```python
from build123d import *
from build123d.topology import SkipClean

# Parameters (mm, degrees)
SKETCH1_W           = 30
SKETCH1_H           = 59
SKETCH1_R           = 7
BOSS_EXTRUDE1_DEPTH = 30
CUT_EXTRUDE1_START  = -14.5
SKETCH2_W           = 30
SKETCH2_H           = 2
CUT_EXTRUDE1_DEPTH  = 4
BOSS_EXTRUDE2_START = 12
SKETCH4_W           = 45
SKETCH4_H           = 59
SKETCH4_R           = 7
BOSS_EXTRUDE2_DEPTH = 12
SKETCH5_R           = 8
CUT_EXTRUDE3_DEPTH  = 8.5
SKETCH8_R           = 10
CUT_EXTRUDE5_DEPTH  = 3.5
BOSS_EXTRUDE4_START = 1.5
BOSS_EXTRUDE4_DEPTH = 1.5
SKETCH12_R          = 6
CUT_EXTRUDE7_DEPTH  = 22
CHAMFER1_SIZE       = 2
MOVE_FACE1_BY       = 1
SKETCH16_W          = 1
SKETCH16_H          = 8
BOSS_EXTRUDE5_DEPTH = 15
SKETCH14_R          = 2.25
CUT_EXTRUDE9_DEPTH  = 70.083283072
BOSS_EXTRUDE6_DEPTH = 20
SKETCH18_R          = 5
CUT_EXTRUDE10_DEPTH = 3
SKETCH19_R          = 2.25
CUT_EXTRUDE11_DEPTH = 81.873357789
SKETCH20_R          = 5
CUT_EXTRUDE12_DEPTH = 7
CHAMFER2_SIZE       = 8
CUT_EXTRUDE13_DEPTH = 2
SKETCH22_R          = 3.3
CUT_EXTRUDE14_DEPTH = 15
CUT_EXTRUDE15_START = -3
CUT_EXTRUDE15_DEPTH = 7
SKETCH24_W          = 8
SKETCH24_H          = 4
SKETCH24_W_2        = 4
SKETCH24_H_2        = 8
BOSS_EXTRUDE7_DEPTH = 4
CUT_EXTRUDE16_START = -31.5
CUT_EXTRUDE16_DEPTH = 31.5


with BuildPart() as part:
    # Sketch1 → Boss-Extrude1 (new body)
    with BuildSketch(Plane.XY):
        with Locations((0, -15)):
            Rectangle(SKETCH1_W, SKETCH1_H)
        Circle(SKETCH1_R, mode=Mode.SUBTRACT)
    extrude(amount=-BOSS_EXTRUDE1_DEPTH)

    # Sketch2 → Cut-Extrude1 (cut, symmetric)
    with BuildSketch(Plane.XZ.offset(44.5).offset(CUT_EXTRUDE1_START)):
        with Locations((0, -29)):
            Rectangle(SKETCH2_W, SKETCH2_H)
    extrude(amount=CUT_EXTRUDE1_DEPTH, both=True, mode=Mode.SUBTRACT)

    # Sketch4 → Boss-Extrude2 (add)
    with BuildSketch(Plane.XY.offset(BOSS_EXTRUDE2_START)):
        with Locations((7.5, -15)):
            Rectangle(SKETCH4_W, SKETCH4_H)
        Circle(SKETCH4_R, mode=Mode.SUBTRACT)
    extrude(amount=-BOSS_EXTRUDE2_DEPTH)

    # Sketch5 → Cut-Extrude3 (cut)
    with BuildSketch(Plane.XY.offset(12)):
        Circle(SKETCH5_R)
    extrude(amount=-CUT_EXTRUDE3_DEPTH, mode=Mode.SUBTRACT)

    # Sketch8 → Cut-Extrude5 (cut)
    with BuildSketch(Plane.XY.offset(12)):
        Circle(SKETCH8_R)
    extrude(amount=-CUT_EXTRUDE5_DEPTH, mode=Mode.SUBTRACT)

    # Sketch11 → Boss-Extrude4 (add)
    with SkipClean():  # the faces are left unmerged after this step: merging them gives an invalid solid
        with BuildSketch(Plane.XY.offset(12).offset(BOSS_EXTRUDE4_START)):
            with BuildLine():
                Line((30, 14.5), (8, 14.5))
                Line((8, 14.5), (8, 6))
                ThreePointArc((8, 6), (10, 0), (8, -6))
                Line((8, -6), (8, -44.5))
                Line((8, -44.5), (30, -44.5))
                Line((30, -44.5), (30, 14.5))
            make_face()
        extrude(amount=-BOSS_EXTRUDE4_DEPTH)

    # Sketch12 → Cut-Extrude7 (cut)
    with SkipClean():  # the faces are left unmerged after this step: merging them gives an invalid solid
        with BuildSketch(Plane(origin=(30, 0, 0), x_dir=(0, 0, -1), z_dir=(1, 0, 0))):
            with Locations((-15, -19)):
                Circle(SKETCH12_R)
        extrude(amount=-CUT_EXTRUDE7_DEPTH, mode=Mode.SUBTRACT)

    # Chamfer1
    # the kernel refuses this chamfer: 2 mm, written as the material it adds along each edge
    with BuildSketch(Plane(origin=(8, -19.052786447, 12), x_dir=(-0.9996219169112968, 0, -0.027495876610586487), z_dir=(0, -1, 0))) as chamfer1_piece_1_section:
        Polygon((CHAMFER1_SIZE * 0.999621916911, -CHAMFER1_SIZE * 0.0274958766106), (-CHAMFER1_SIZE * 0.0274958766106, -CHAMFER1_SIZE * 0.999621916911), (0, 0), align=None)
    chamfer1_piece_1 = extrude(amount=25.447213553, mode=Mode.PRIVATE)
    chamfer1_piece_1 = chamfer1_piece_1 - Plane(origin=(7.298262976, -19, 15), x_dir=(0, 0, -1), z_dir=(1, 0, 0)) * Cylinder(6, 59, mode=Mode.PRIVATE)
    chamfer1_piece_1 = split(chamfer1_piece_1, bisect_by=Plane(origin=(7.298262976, -34.489945177, 13.5), z_dir=(0, 0, -1)), keep=Keep.TOP, mode=Mode.PRIVATE)
    add(chamfer1_piece_1)
    with BuildSketch(Plane(origin=(8, 14.5, 12), x_dir=(-0.9996219169112968, 0, -0.027495876610586487), z_dir=(0, -1, 0))) as chamfer1_piece_2_section:
        Polygon((CHAMFER1_SIZE * 0.999621916911, -CHAMFER1_SIZE * 0.0274958766106), (-CHAMFER1_SIZE * 0.0274958766106, -CHAMFER1_SIZE * 0.999621916911), (0, 0), align=None)
    chamfer1_piece_2 = extrude(amount=13.643365976, mode=Mode.PRIVATE)
    chamfer1_piece_2 = chamfer1_piece_2 - Plane(origin=(0, 0, 12.610971558), x_dir=(1, 0, 0), z_dir=(0, 0, 1)) * Cylinder(10, 36, mode=Mode.PRIVATE)
    chamfer1_piece_2 = split(chamfer1_piece_2, bisect_by=Plane(origin=(7.329577736, 10.634975656, 13.5), z_dir=(0, 0, -1)), keep=Keep.TOP, mode=Mode.PRIVATE)
    add(chamfer1_piece_2)
    with BuildSketch(Plane(origin=(8, -0.856634024, 12), x_dir=(-0.9996219169112968, 0, -0.027495876610586487), z_dir=(0, -1, 0))) as chamfer1_piece_3_section:
        Polygon((CHAMFER1_SIZE * 0.999621916911, -CHAMFER1_SIZE * 0.0274958766106), (-CHAMFER1_SIZE * 0.0274958766106, -CHAMFER1_SIZE * 0.999621916911), (0, 0), align=None)
    chamfer1_piece_3 = extrude(amount=18.090579529, mode=Mode.PRIVATE)
    chamfer1_piece_3 = chamfer1_piece_3 - Plane(origin=(7.328722349, -19, 15), x_dir=(0, 0, -1), z_dir=(1, 0, 0)) * Cylinder(6, 45, mode=Mode.PRIVATE)
    chamfer1_piece_3 = chamfer1_piece_3 - Plane(origin=(0, 0, 12.602221716), x_dir=(1, 0, 0), z_dir=(0, 0, 1)) * Cylinder(10, 45, mode=Mode.PRIVATE)
    chamfer1_piece_3 = split(chamfer1_piece_3, bisect_by=Plane(origin=(7.328722349, -10.144229593, 13.5), z_dir=(0, 0, -1)), keep=Keep.TOP, mode=Mode.PRIVATE)
    add(chamfer1_piece_3)

    # Move Face1: a face moved outward by 1.0
    extrude(part.faces().sort_by_distance((8, -19, 10.769879029))[0], amount=MOVE_FACE1_BY, dir=(1, 0, 0))

    # Sketch16 → Boss-Extrude5 (add)
    with BuildSketch(Plane(origin=(30, 0, 0), x_dir=(0, 0, -1), z_dir=(1, 0, 0))):
        with Locations((0.5, 0)):
            Rectangle(SKETCH16_W, SKETCH16_H)
        with Locations((0.5, -30)):
            Rectangle(SKETCH16_W, SKETCH16_H)
    extrude(amount=-BOSS_EXTRUDE5_DEPTH)

    # Sketch14 → Cut-Extrude9 (cut, through all)
    with BuildSketch(Plane.XY.offset(13.5)):
        with Locations((22.5, 0)):
            Circle(SKETCH14_R)
        with Locations((22.5, -30)):
            Circle(SKETCH14_R)
    extrude(amount=-CUT_EXTRUDE9_DEPTH, mode=Mode.SUBTRACT)

    # Sketch18 → Cut-Extrude10 (cut)
    with BuildSketch(Plane.XY.offset(13.5)):
        with Locations((22.5, 0)):
            Circle(SKETCH18_R)
    extrude(amount=-CUT_EXTRUDE10_DEPTH, mode=Mode.SUBTRACT)

    # Sketch21 → Cut-Extrude13 (cut)
    with BuildSketch(Plane(origin=(15, 0, 0), x_dir=(0, 0, -1), z_dir=(1, 0, 0))):
        Polygon((0, 9), (10, 9), (10, -9), (0, -9), (0, -4), (1, -4), (1, 4), (0, 4), align=None)
        Polygon((0, -21), (10, -21), (10, -39), (0, -39), (0, -34), (1, -34), (1, -26), (0, -26), align=None)
    extrude(amount=-CUT_EXTRUDE13_DEPTH, mode=Mode.SUBTRACT)

    # Sketch22 → Cut-Extrude14 (cut)
    with BuildSketch(Plane(origin=(0, 0, -28), x_dir=(-1, 0, 0), z_dir=(0, 0, -1))):
        with Locations((-0.001598667, -30)):
            Circle(SKETCH22_R)
    extrude(amount=-CUT_EXTRUDE14_DEPTH, mode=Mode.SUBTRACT)

    # Sketch23 → Cut-Extrude15 (cut)
    with BuildSketch(Plane(origin=(0, 0, -28), x_dir=(-1, 0, 0), z_dir=(0, 0, -1)).offset(CUT_EXTRUDE15_START)):
        Polygon((-5.101598667, -32.944486373), (-5.101598667, -44.5), (5.098401333, -44.5), (5.098401333, -32.944486373), (5.098401333, -27.055513627), (-0.001598667, -24.111027254), (-5.101598667, -27.055513627), align=None)
    extrude(amount=-CUT_EXTRUDE15_DEPTH, mode=Mode.SUBTRACT)

    # Sketch24 → Boss-Extrude7 (add)
    with BuildSketch(Plane(origin=(15, 0, 0), x_dir=(0, 0, -1), z_dir=(1, 0, 0))):
        with Locations((15, 12.5)):
            Rectangle(SKETCH24_W, SKETCH24_H)
        with Locations((28, 0)):
            Rectangle(SKETCH24_W_2, SKETCH24_H_2)
    extrude(amount=BOSS_EXTRUDE7_DEPTH)

    # Sketch25 → Cut-Extrude16 (cut)
    with BuildSketch(Plane(origin=(0, 0, -30), x_dir=(-1, 0, 0), z_dir=(0, 0, -1)).offset(CUT_EXTRUDE16_START)):
        with BuildLine():
            Line((-8.191520443, 5.735764364), (-12.207745888, 0))
            Line((-12.207745888, 0), (-8.191520443, -5.735764364))
            ThreePointArc((-8.191520443, -5.735764364), (10, 0), (-8.191520443, 5.735764364))
        make_face()
    extrude(amount=CUT_EXTRUDE16_DEPTH, mode=Mode.SUBTRACT)


with BuildPart() as body_2:
    # Sketch17 → Boss-Extrude6 (new body)
    with BuildSketch(Plane(origin=(30, 0, 0), x_dir=(0, 0, -1), z_dir=(1, 0, 0))):
        with BuildLine():
            Line((-16.5, -13.190524981), (-16.5, -9.5))
            Line((-16.5, -9.5), (-30.5, -9.5))
            Line((-30.5, -9.5), (-30.5, -44.5))
            Line((-30.5, -44.5), (-13.5, -44.5))
            Line((-13.5, -44.5), (-13.5, -40.5))
            Line((-13.5, -40.5), (-16.5, -40.5))
            Line((-16.5, -40.5), (-16.5, -24.809475019))
            ThreePointArc((-16.5, -24.809475019), (-21, -19), (-16.5, -13.190524981))
        make_face()
    extrude(amount=-BOSS_EXTRUDE6_DEPTH)

    # Sketch19 → Cut-Extrude11 (cut, through all)
    with BuildSketch(Plane.XY.offset(30.5)):
        with Locations((22.5, -30)):
            Circle(SKETCH19_R)
    extrude(amount=-CUT_EXTRUDE11_DEPTH, mode=Mode.SUBTRACT)

    # Sketch20 → Cut-Extrude12 (cut)
    with BuildSketch(Plane.XY.offset(30.5)):
        with Locations((22.5, -30)):
            Circle(SKETCH20_R)
    extrude(amount=-CUT_EXTRUDE12_DEPTH, mode=Mode.SUBTRACT)

    # Chamfer2
    chamfer2_edges = [body_2.edges().sort_by_distance(p)[0] for p in [
        (20, -9.5, 30.5),
    ]]
    chamfer(chamfer2_edges, length=CHAMFER2_SIZE)


solid = body_2.part
```
Check sheet for the modelled part. Datum: model origin and axes. Units: mm. A direction names the side the tool comes from. Give positions to 0.01 mm unless a question says otherwise; leave off trailing zeros. Order: outer loops, then holes, each group sorted by start corner. A loop starts at its lowest first (then second) coordinate and runs counter-clockwise, first axis right, second up. Notation, with made-up numbers: M -40,28 L 0,28 A30 cw 0,55 Z; hole C -34,85 d8. An arc over 180 degrees is marked long. Answer in a Markdown table with one row per item.
1) Thickness scan on L1, parallel to Y at x = 22.5, z = 18.75; L2, parallel to Z at x = 18, y = -28; L3, parallel to Y at x = 22.5, z = 21.75. Record the ranges inside material, lowest first. Write a range as [from, to].
Filled sheet:
| item | result |
|---|---|
| L1 | y = [-44.5, -32.25], [-27.75, -23.68], [-14.32, -9.5] |
| L2 | z = [16.5, 23.5] |
| L3 | y = [-44.5, -32.25], [-27.75, -9.5] |
2) Release check for a two-part mould opening along X. For faces 4 (the flat face through (10, -31, 24)), 5 (the flat face through (20, -14, 27)), 6 (the flat face through (24, -32, 23.5)) record: +X half, -X half, draft (parallel to the pull), parting line (faces both ways), or undercut.
Filled sheet:
| item | result |
|---|---|
| face 4 | -X half |
| face 5 | draft |
| face 6 | undercut |
3) Cross-section at A-A, the plane y = -30. Enter the section's corners in (x, z), plus the area to 4 significant figures.
Filled sheet:
| item | result |
|---|---|
| outline | M 10,16.5 L 20.25,16.5 L 20.25,23.5 L 17.5,23.5 L 17.5,30.5 L 10,30.5 Z; M 24.75,16.5 L 30,16.5 L 30,30.5 L 27.5,30.5 L 27.5,23.5 L 24.75,23.5 Z |
| area | 178.5 mm2 |
4) Cross-section at C-C, the plane x = 22.5. Enter the section's corners in (y, z), plus the area to 3 significant figures.
Filled sheet:
| item | result |
|---|---|
| outline | M -44.5,13.5 L -40.5,13.5 L -40.5,16.5 L -32.25,16.5 L -32.25,23.5 L -35,23.5 L -35,30.5 L -44.5,30.5 Z; M -27.75,16.5 L -24.81,16.5 A6 cw -13.19,16.5 L -9.5,16.5 L -9.5,22.5 L -17.5,30.5 L -25,30.5 L -25,23.5 L -27.75,23.5 Z |
| area | 330 mm2 |
5) Gauge pin test, flat ends, axial feed: P1, Ø5, axis at x = 22.5, y = -30, coming from the +Z side; P2, Ø0.9, axis at x = 17, z = 15, coming from the +Y side; P3, Ø2, axis at x = 22, y = -34, coming from the -Z side. Record the tip position at first contact, or that the pin passes through.
Filled sheet:
| item | result |
|---|---|
| P1 | stops at z = 23.5 |
| P2 | stops at y = -40.5 |
| P3 | stops at z = 16.5 |
6) Cross-section at D-D, the plane z = 14.5. Enter the section's corners in (x, y), plus the area to 3 significant figures.
Filled sheet:
| item | result |
|---|---|
| outline | M 10,-44.5 L 30,-44.5 L 30,-40.5 L 10,-40.5 Z |
| area | 80.0 mm2 |
7) Access from +Z, -Z, +X, -X, +Y, -Y to the whole of each face (thin tool, end or side, straight path). Record for faces 1 (the flat face through (20, -40.5, 15)), 2 (the cylindrical face through (21.42, -34.88, 27.05)), 3 (the cylindrical face through (20, -19, 21)).
Filled sheet:
| item | result |
|---|---|
| face 1 | -Z, +X, -X, +Y |
| face 2 | +Z |
| face 3 | -Z, +X, -X |
8) Cross-section at B-B, the plane z = 17.75. Enter the section's corners in (x, y).
Filled sheet:
| item | result |
|---|---|
| outline | M 10,-44.5 L 30,-44.5 L 30,-24.33 L 10,-24.33 Z; M 10,-13.67 L 30,-13.67 L 30,-9.5 L 10,-9.5 Z; hole C 22.5,-30 d4.5 |
